from build123d import *

# Parameters (mm, degrees)
SKETCH1_W           = 139.7
SKETCH1_H           = 139.7
BOSS_EXTRUDE1_DEPTH = 12.7
SKETCH2_W           = 136.7
SKETCH2_H           = 136.7
CUT_EXTRUDE1_DEPTH  = 0.3
CUT_EXTRUDE2_START  = -22.4
CUT_EXTRUDE2_DEPTH  = 125.396102867
SKETCH18_W          = 10.16
SKETCH18_H          = 4.875
CUT_EXTRUDE6_DEPTH  = 20
FILLET1_R           = 1
CIRPATTERN1_COUNT   = 4
SKETCH19_W          = 100
SKETCH19_H          = 100
CUT_EXTRUDE8_DEPTH  = 3.5
SKETCH20_W          = 96
SKETCH20_H          = 96
CUT_EXTRUDE9_DEPTH  = 18.6
SKETCH21_W          = 30
SKETCH21_H          = 10
CUT_EXTRUDE10_DEPTH = 102.290695525
FILLET2_R           = 1.5


with BuildPart() as part:
    # Sketch1 → Boss-Extrude1 (new, symmetric)
    with BuildSketch(Plane(origin=(0, 0, 0), x_dir=(1, 0, 0), z_dir=(0, 1, 0))):
        Rectangle(SKETCH1_W, SKETCH1_H)
    extrude(amount=BOSS_EXTRUDE1_DEPTH, both=True)

    # Sketch2 → Cut-Extrude1 (cut)
    with BuildSketch(Plane(origin=(0, 12.7, 0), x_dir=(1, 0, 0), z_dir=(0, 1, 0))):
        Rectangle(SKETCH2_W, SKETCH2_H)
    extrude(amount=-CUT_EXTRUDE1_DEPTH, mode=Mode.SUBTRACT)

    # Sketch4 → Cut-Extrude2 (cut)
    with BuildSketch(Plane(origin=(0, 12.7, 0), x_dir=(1, 0, 0), z_dir=(0, 1, 0)).offset(CUT_EXTRUDE2_START)):
        Polygon((-43.283333333, -69.85), (-50.500211698, -57.35), (-6.066454968, -57.35), (-13.283333333, -69.85), align=None)
        Polygon((43.283333333, -69.85), (36.066454968, -57.35), (20.500211698, -57.35), (13.283333333, -69.85), align=None)
    cut_extrude2 = extrude(amount=CUT_EXTRUDE2_DEPTH, mode=Mode.SUBTRACT)

    # Sketch18 → Cut-Extrude6 (cut)
    with BuildSketch(Plane.XY.offset(57.35)):
        with Locations((28.283333333, 9.9625)):
            Rectangle(SKETCH18_W, SKETCH18_H)
        with Locations((-28.283333333, 9.9625)):
            Rectangle(SKETCH18_W, SKETCH18_H)
    cut_extrude6 = extrude(amount=-CUT_EXTRUDE6_DEPTH, mode=Mode.SUBTRACT)

    # Fillet1
    fillet1_edges = [part.edges().sort_by_distance(p)[0] for p in [
        (-68.35, 12.55, -68.35),
        (-68.35, 12.55, 68.35),
        (68.35, 12.55, 68.35),
        (68.35, 12.55, -68.35),
    ]]
    fillet(fillet1_edges, radius=FILLET1_R)

    # CirPattern1: Cut-Extrude2, Cut-Extrude6 ×4 about axis
    cirpattern1_axis = Axis((0, 0, 0), (0, 1, 0))
    add([cut_extrude2.rotate(cirpattern1_axis, i * 360 / CIRPATTERN1_COUNT) for i in range(1, CIRPATTERN1_COUNT)], mode=Mode.SUBTRACT)
    add([cut_extrude6.rotate(cirpattern1_axis, i * 360 / CIRPATTERN1_COUNT) for i in range(1, CIRPATTERN1_COUNT)], mode=Mode.SUBTRACT)

    # Sketch19 → Cut-Extrude8 (cut)
    with BuildSketch(Plane(origin=(0, 12.4, 0), x_dir=(1, 0, 0), z_dir=(0, 1, 0))):
        Rectangle(SKETCH19_W, SKETCH19_H)
    extrude(amount=-CUT_EXTRUDE8_DEPTH, mode=Mode.SUBTRACT)

    # Sketch20 → Cut-Extrude9 (cut)
    with BuildSketch(Plane(origin=(0, 8.9, 0), x_dir=(1, 0, 0), z_dir=(0, 1, 0))):
        Rectangle(SKETCH20_W, SKETCH20_H)
    extrude(amount=-CUT_EXTRUDE9_DEPTH, mode=Mode.SUBTRACT)

    # Sketch21 → Cut-Extrude10 (cut, through all)
    with BuildSketch(Plane(origin=(0, -9.7, 0), x_dir=(1, 0, 0), z_dir=(0, 1, 0))):
        with Locations((-28, 38)):
            Rectangle(SKETCH21_W, SKETCH21_H)
    extrude(amount=-CUT_EXTRUDE10_DEPTH, mode=Mode.SUBTRACT)

    # Fillet2
    fillet2_edges = [part.edges().sort_by_distance(p)[0] for p in [
        (50, 10.65, 50),
        (-50, 10.65, -50),
        (-50, 10.65, 50),
        (50, 10.65, -50),
        (48, -0.4, -48),
        (48, -0.4, 48),
        (-48, -0.4, 48),
        (-48, -0.4, -48),
    ]]
    fillet(fillet2_edges, radius=FILLET2_R)


solid = part.part
Part model, mm, in its own coordinate system. A direction names the side the tool comes from. Give positions to 0.01 mm unless a question says otherwise; leave off trailing zeros. Order: outer loops, then holes, each group sorted by start corner. A loop starts at its lowest first (then second) coordinate and runs counter-clockwise, first axis right, second up. Notation, with made-up numbers: (88, 35) - (122, 35) arc R17 ccw to (122, 47) - close; hole circle Ø6 at (46, 48). An arc over 180 degrees is marked (long way). Use a Markdown table: item, result.
1) Saw through at B-B on x = -2.5. List the corners of the cut face in (y, z), plus the area to 3 significant figures.
Checked values:
| item | result |
|---|---|
| outline | (-12.7, -69.85) - (12.7, -69.85) - (12.7, -68.35) - (12.4, -68.35) - (12.4, -50) - (8.9, -50) - (8.9, -48) - (-9.7, -48) - (-9.7, 48) - (8.9, 48) - (8.9, 50) - (12.4, 50) - (12.4, 68.35) - (12.7, 68.35) - (12.7, 69.85) - (-12.7, 69.85) - close |
| area | 1,370 mm² |
2) Flat gauge pins, fed straight in: P1, Ø12, axis at x = 33.5, y = -2, coming from the -Z side; P2, Ø4, axis at x = 29.5, z = -62.5, coming from the +Y side; P3, Ø3, axis at x = 37.5, y = 10.5, coming from the +Z side. Where does each tip first touch, or does it go through?
Checked values:
| item | result |
|---|---|
| P1 | z = -57.35 |
| P2 | y = -9.7 |
| P3 | z = 62.43 |
3) Saw through at C-C on y = 10.5. Count the separate pieces of the cut face and the enclosed holes in it, plus the area to 3 significant figures.
Checked values:
| item | result |
|---|---|
| separate pieces | 8 |
| enclosed holes | 0 |
| area | 5,920 mm² |
4) Two-plate mould, pull along Z, no slides. Class faces 1 (the flat face through (39.725, 1.343, 63.687)), 2 (the flat face through (-43, -11, -38)), 3 (the flat face through (-28, -1, -57.35)): +Z half, -Z half, draft (parallel to the pull), parting line (faces both ways), or undercut.
Checked values:
| item | result |
|---|---|
| face 1 | +Z half |
| face 2 | undercut |
| face 3 | -Z half |
5) Probe L1, parallel to Z at x = -51, y = 10; L2, parallel to Z at x = 31, y = 6.25. List the from-to ranges inside material, lowest first. Write a range as from..to.
Checked values:
| item | result |
|---|---|
| L1 | -69.85..-33.36, -23.2..23.2, 33.36..69.85 |
| L2 | -57.35..-48, 48..57.35 |
6) Saw through at D-D on x = -55. List the corners of the cut face in (y, z) (3 decimals).
Checked values:
| item | result |
|---|---|
| outline | (-12.7, -69.85) - (12.7, -69.85) - (12.7, -68.35) - (12.4, -68.35) - (12.4, -33.363) - (7.525, -33.363) - (7.525, -23.203) - (12.4, -23.203) - (12.4, 23.203) - (7.525, 23.203) - (7.525, 33.363) - (12.4, 33.363) - (12.4, 68.35) - (12.7, 68.35) - (12.7, 69.85) - (-12.7, 69.85) - close |
7) Saw through at A-A on z = -27. List the corners of the cut face in (x, y) (3 decimals).
Checked values:
| item | result |
|---|---|
| outline | (-69.85, -12.7) - (69.85, -12.7) - (69.85, -9.7) - (57.35, -9.7) - (57.35, 7.525) - (48, 7.525) - (48, -9.7) - (-48, -9.7) - (-48, 7.525) - (-57.35, 7.525) - (-57.35, -9.7) - (-69.85, -9.7) - close |
8) 3-axis set-ups, long thin cutter, end or side, ignore diameter. For faces 4 (the flat face through (-41, 11, -50)), 5 (the flat face through (-13, -11, -38)), 6 (the flat face through (-23.203, 10, -54)), 7 (the flat face through (28, -9.7, 65)): which of +Z, -Z, +X, -X, +Y, -Y reach the whole face in a straight line?
Checked values:
| item | result |
|---|---|
| face 4 | +Y |
| face 5 | +Y, -Y |
| face 6 | +Z, -Z, +Y |
| face 7 | +Z, +Y |
